```python
from build123d import *

# Parameters (mm, degrees)
F0_W     = 203.2
F0_H     = 12.7
F1_DEPTH = 9.525
F2_W     = 19.05
F2_H     = 6.35
F3_DEPTH = 25.4
F4_W     = 6.35
F4_H     = 6.35
F5_DEPTH = 6.35
F7_DEPTH = 25.4


with BuildPart() as f1:
    # F0 (on Top) → F1 (new body)
    with BuildSketch(Plane.XY):
        Rectangle(F0_W, F0_H)
    extrude(amount=F1_DEPTH)

    # F2 (on face) → F3 (cut)
    with BuildSketch(Plane(origin=(0, 6.35, 0), x_dir=(-1, 0, 0), z_dir=(0, 1, 0))):
        with Locations((-92.075, 3.175)):
            Rectangle(F2_W, F2_H)
        with Locations((92.075, 3.175)):
            Rectangle(F2_W, F2_H)
    extrude(amount=-F3_DEPTH, mode=Mode.SUBTRACT)

    # F4 (on face) → F5 (join, through all)
    with BuildSketch(Plane(origin=(0, 0, 0), x_dir=(1, 0, 0), z_dir=(0, 0, -1))):
        with Locations((-92.075, 0)):
            Rectangle(F4_W, F4_H)
        with Locations((92.075, 0)):
            Rectangle(F4_W, F4_H)
    extrude(amount=-F5_DEPTH)

    # F6 (on face) → F7 (cut)
    with BuildSketch(Plane(origin=(0, 6.35, 0), x_dir=(-1, 0, 0), z_dir=(0, 1, 0))):
        Polygon((-82.55, 0), (82.55, 0), (76.2, 6.35), (-76.2, 6.35), align=None)
    extrude(amount=-F7_DEPTH, mode=Mode.SUBTRACT)


solid = f1.part
```
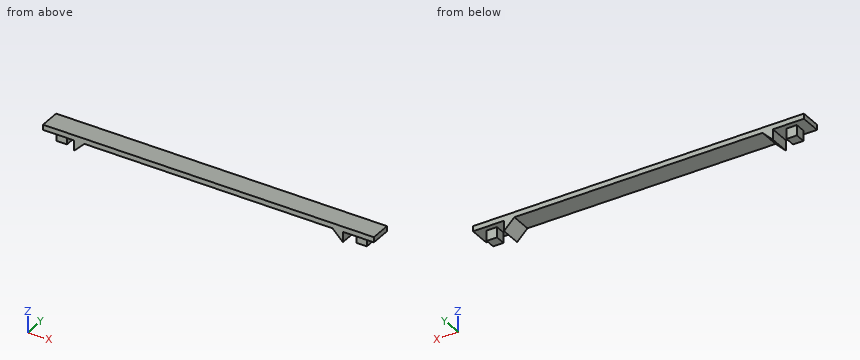
Build history of the part. All positions in model axes, mm. Round coordinates to 2 decimals unless told otherwise and drop trailing zeros. Loops run counter-clockwise (first coordinate to the right, second up) from the corner with the lowest first, then second, coordinate; pieces in that order, holes last.
Item 1: Pin check, flat tips, straight feed: P1, Ø1.9, axis at x = -93, z = 1.5, coming from the -Y side (3 decimals); P2, Ø2, axis at y = 4, z = 5, coming from the -X side; P3, Ø2, axis at y = -4.5, z = 5, coming from the -X side. Stop position of each tip, or through.
Item 2: Saw through at C-C (x = -49.5). List the corners of the cut face in (y, z) (3 decimals).
Item 3: Drill centre lines: line 1 along X through (y, z) = (-1, 4); line 2 along X through (y, z) = (-0.75, 4.5); line 3 along Z through (x, y) = (-60, -3.75) (3 decimals). Where is each one in solid material? Low to high.
Item 4: Saw through at A-A (z = 1.5). List the corners of the cut face in (x, y) (3 decimals), then the cut area to 3 significant figures.
Item 5: Saw through at B-B (y = 0). List the corners of the cut face in (x, z) (3 decimals).
Worked answers:
1. P1: stops at y = -3.175
1. P2: stops at x = -95.25
1. P3: stops at x = -82.55
2. outline: (-6.35, 6.35) - (6.35, 6.35) - (6.35, 9.525) - (-6.35, 9.525) - close
3. line 1: x = -95.25 to -88.9, -82.55 to -78.55, 78.55 to 82.55, 88.9 to 95.25
3. line 2: x = -95.25 to -88.9, -82.55 to -78.05, 78.05 to 82.55, 88.9 to 95.25
3. line 3: z = 6.35 to 9.525
4. outline: (-95.25, -3.175) - (-88.9, -3.175) - (-88.9, 3.175) - (-95.25, 3.175) - close; (-82.55, -6.35) - (-81.05, -6.35) - (-81.05, 6.35) - (-82.55, 6.35) - close; (81.05, -6.35) - (82.55, -6.35) - (82.55, 6.35) - (81.05, 6.35) - close; (88.9, -3.175) - (95.25, -3.175) - (95.25, 3.175) - (88.9, 3.175) - close
4. area: 119 mm2
5. outline: (-101.6, 6.35) - (-95.25, 6.35) - (-95.25, 0) - (-88.9, 0) - (-88.9, 6.35) - (-82.55, 6.35) - (-82.55, 0) - (-76.2, 6.35) - (76.2, 6.35) - (82.55, 0) - (82.55, 6.35) - (88.9, 6.35) - (88.9, 0) - (95.25, 0) - (95.25, 6.35) - (101.6, 6.35) - (101.6, 9.525) - (-101.6, 9.525) - close
